from build123d import *

# Parameters (mm, degrees)
SKETCH1_W           = 71.272685497
SKETCH1_H           = 48.354613482
BOSS_EXTRUDE1_DEPTH = 12.7
SKETCH2_W           = 61.031917372
SKETCH2_H           = 39.617209522
CUT_EXTRUDE1_DEPTH  = 6.35
BOSS_EXTRUDE2_DEPTH = 48.354613
FILLET1_R           = 2.54
SKETCH5_R           = 7.62
CUT_EXTRUDE2_DEPTH  = 2.54
CUT_EXTRUDE3_DEPTH  = 6.35
CUT_REVOLVE1_ANGLE  = 180


with BuildPart() as part:
    # Sketch1 → Boss-Extrude1 (new body)
    with BuildSketch(Plane(origin=(0, 0, 0), x_dir=(1, 0, 0), z_dir=(0, 1, 0))):
        with Locations((0.881464309, -2.644392925)):
            Rectangle(SKETCH1_W, SKETCH1_H)
    extrude(amount=-BOSS_EXTRUDE1_DEPTH)

    # Sketch2 → Cut-Extrude1 (cut)
    with BuildSketch(Plane(origin=(0, 0, 0), x_dir=(1, 0, 0), z_dir=(0, 1, 0))):
        with Locations((0.488861331, -2.573010565)):
            Rectangle(SKETCH2_W, SKETCH2_H)
    extrude(amount=-CUT_EXTRUDE1_DEPTH, mode=Mode.SUBTRACT)

    # Sketch4 → Boss-Extrude2 (add)
    with BuildSketch(Plane.XY.offset(26.821699666)):
        Polygon((-34.75487844, -12.7), (-34.75487844, -26.729663637), (-49.514481499, -26.729663637), (-34.75487844, 0), align=None)
    extrude(amount=-BOSS_EXTRUDE2_DEPTH)

    # Fillet1
    fillet1_edges = [part.edges().sort_by_distance(p)[0] for p in [
        (-34.75487844, 0, 2.644392925),
    ]]
    fillet(fillet1_edges, radius=FILLET1_R)

    # Sketch5 → Cut-Extrude2 (cut)
    with BuildSketch(Plane(origin=(0, 0, -21.532913816), x_dir=(-1, 0, 0), z_dir=(0, 0, -1))):
        with Locations((-13.922709082, -12.7)):
            Circle(SKETCH5_R)
    extrude(amount=-CUT_EXTRUDE2_DEPTH, mode=Mode.SUBTRACT)

    # Sketch7 → Cut-Extrude3 (cut)
    with BuildSketch(Plane(origin=(0, -6.35, 0), x_dir=(1, 0, 0), z_dir=(0, 1, 0))):
        with BuildLine():
            Line((-25.109899832, 14.028476446), (-25.109899832, 7.738453376))
            ThreePointArc((-25.109899832, 7.738453376), (-26.574699725, 6.273653483), (-28.039499618, 7.738453376))
            Line((-28.039499618, 7.738453376), (-28.039499618, 14.028476446))
            ThreePointArc((-28.039499618, 14.028476446), (-26.574699725, 15.493276339), (-25.109899832, 14.028476446))
        make_face()
        with BuildLine():
            Line((-25.435843167, -12.298214097), (-25.435843167, -18.588237167))
            ThreePointArc((-25.435843167, -18.588237167), (-26.90064306, -20.05303706), (-28.365442953, -18.588237167))
            Line((-28.365442953, -18.588237167), (-28.365442953, -12.298214097))
            ThreePointArc((-28.365442953, -12.298214097), (-26.90064306, -10.833414204), (-25.435843167, -12.298214097))
        make_face()
    extrude(amount=-CUT_EXTRUDE3_DEPTH, mode=Mode.SUBTRACT)

    # Sketch9 → Cut-Revolve1 (revolve, cut)
    with BuildSketch(Plane(origin=(-34.75487844, 0, 0), x_dir=(0, 0, -1), z_dir=(1, 0, 0))):
        Polygon((-2.644392925, -26.729663637), (-2.644392925, -13.548328756), (-0.340047454, -13.548328756), (3.5393378, -26.729663637), align=None)
    revolve(axis=Axis((-34.75487844, -26.729663637, 2.644392925), (0, 1, 0)), revolution_arc=CUT_REVOLVE1_ANGLE, mode=Mode.SUBTRACT)


solid = part.part
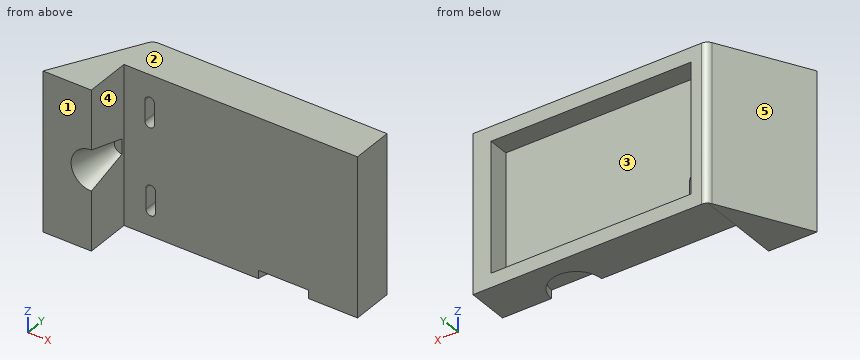
Source: CAD feature listing. Evaluate the final solid. Frame: model axes, mm. Face numbers are marked on the shaded views. A direction names the side the tool comes from. Coordinates: 2 decimals unless noted, no trailing zeros. Loops run counter-clockwise (first coordinate to the right, second up) from the corner with the lowest first, then second, coordinate; pieces in that order, holes last. Notation, with made-up numbers: (43.25, 74.25) - (58.25, 74.25) arc R22 ccw to (58.25, 108.25) - close; hole circle Ø9 at (68.25, 84). An arc over 180 degrees is marked (long way). One line per item, written item: value. Start each with the question number.
1. Section D-D (y = -18.5). Return the cut outline in (x, z), and give its area (3 significant figures).
2. Mould query, pull axis Z, two halves, no side actions, for the marked faces 1, 2 and 3. Classes: pulls with the +Z half, pulls with the -Z half, needs draft (parallel to the pull), parting line crosses it, or undercut.
3. Contact query for flat-ended pins moving along their axis: P1, Ø8, axis at x = 0.5, z = 10.5, coming from the +Y side; P2, Ø3, axis at y = -4, z = 3, coming from the -X side; P3, Ø1.5, axis at x = 3.5, z = 8.5, coming from the -Y side. Output: stop coordinate, or through.
4. Section B-B (y = -9.75). Return the cut outline in (x, z), and give its area (3 significant figures).
5. Section C-C (x = -7.5). Return the cut outline in (y, z), and give its area (3 significant figures).
6. Ray query, L1, parallel to Z at x = -17.5, y = -1.25; L2, parallel to Y at x = 24, z = 15; L3, parallel to Y at x = -31.5, z = 21.5. Return the intervals inside material, ascending.
7. Section A-A (z = -11.5). Return the cut outline in (x, y).
8. Set-up query: the marked faces 4 and 5. Return all of +Z, -Z, +X, -X, +Y, -Y with unobstructed straight access to the full face (end or side cutting, diameter ignored); none if empty.
Verdict:
1. outline: (-44.97, -21.53) - (-34.75, -21.53) - (-34.75, -1.12) arc R3.76 cw to (-34.75, 6.41) - (-34.75, 26.82) - (-44.97, 26.82) - close
1. area: 472 mm2
2. face 1: needs draft
2. face 2: pulls with the +Z half
2. face 3: undercut
3. P1: stops at y = -6.35
3. P2: stops at x = -37.79
3. P3: stops at y = -12.7
4. outline: (-40.14, -21.53) - (6.9, -21.53) - (6.9, -18.99) - (20.95, -18.99) - (20.95, -21.53) - (36.52, -21.53) - (36.52, 26.82) - (-40.14, 26.82) - close; hole (-28.37, 12.3) arc R1.46 ccw to (-25.44, 12.3) - (-25.44, 18.59) arc R1.46 ccw to (-28.37, 18.59) - close; hole (-28.04, -14.03) arc R1.46 ccw to (-25.11, -14.03) - (-25.11, -7.74) arc R1.46 ccw to (-28.04, -7.74) - close
4. area: 3,620 mm2
5. outline: (-12.7, -21.53) - (0, -21.53) - (0, -17.24) - (-6.35, -17.24) - (-6.35, 22.38) - (0, 22.38) - (0, 26.82) - (-12.7, 26.82) - close
5. area: 363 mm2
6. L1: z = -21.53 to -17.24, 22.38 to 26.82
6. L2: y = -12.7 to -6.35
6. L3: y = -12.7 to 0
7. outline: (-49.51, -26.73) - (-34.75, -26.73) - (-34.75, -12.7) - (-28.04, -12.7) - (-28.04, -6.35) - (-30.03, -6.35) - (-30.03, 0) - (-33.26, 0) arc R2.54 ccw to (-35.48, -1.31) - close; (-25.11, -12.7) - (36.52, -12.7) - (36.52, 0) - (31, 0) - (31, -6.35) - (-25.11, -6.35) - close
8. face 4: +Z, -Z, +X, -Y
8. face 5: +Z, -Z, -X, +Y
